Geometry: final body of the model. Coordinates: model frame, mm. Face numbers are marked on the shaded views. Give positions to 0.01 mm unless a question says otherwise; leave off trailing zeros. Put each result on its own line as item: value. Start each with the question number.
1. First-contact query: P1, Ø1.7, axis at x = 0.5, z = -20, coming from the -Y side; P2, Ø3.5, axis at x = 0, z = -19.05, coming from the +Y side. Flat tips, straight axial feed; report the tip coordinate or a pass-through.
2. Ray query, line 1 along Z through (x, y) = (0, -515.75); line 2 along X through (y, z) = (-19, -19); line 3 along X through (y, z) = (-352, -40.5). Return the intervals inside material, ascending. Write a range as from..to.
3. Mould query, pull axis Z, two halves, no side actions, for the marked faces 1, 2 and 3. Classes: pulls with the +Z half, pulls with the -Z half, needs draft (parallel to the pull), parting line crosses it, or undercut.
from build123d import *

# Parameters (mm, degrees)
F0_W     = 38.1
F0_H     = 88.9
F1_DEPTH = 533.4
F2_R     = 5.08
F3_R     = 2.8575
F4_DEPTH = 25.4
F5_R     = 2.8575
F6_DEPTH = 25.4


with BuildPart() as f1:
    # F0 (on Front) → F1 (new body)
    with BuildSketch(Plane.XZ):
        Rectangle(F0_W, F0_H)
    extrude(amount=F1_DEPTH)

    # F2
    f2_edges = [f1.edges().sort_by_distance(p)[0] for p in [
        (19.05, -266.7, 44.45),
        (-19.05, -266.7, 44.45),
        (19.05, -266.7, -44.45),
        (-19.05, -266.7, -44.45),
    ]]
    fillet(f2_edges, radius=F2_R)

    # F3 (on face) → F4 (cut)
    with BuildSketch(Plane.XZ.offset(533.4)):
        with Locations((0, -19.05)):
            Circle(F3_R)
        with Locations((0, 19.05)):
            Circle(F3_R)
    extrude(amount=-F4_DEPTH, mode=Mode.SUBTRACT)

    # F5 (on face) → F6 (cut)
    with BuildSketch(Plane(origin=(0, 0, 0), x_dir=(-1, 0, 0), z_dir=(0, 1, 0))):
        with Locations((0, 19.05)):
            Circle(F5_R)
        with Locations((0, -19.05)):
            Circle(F5_R)
    extrude(amount=-F6_DEPTH, mode=Mode.SUBTRACT)


solid = f1.part
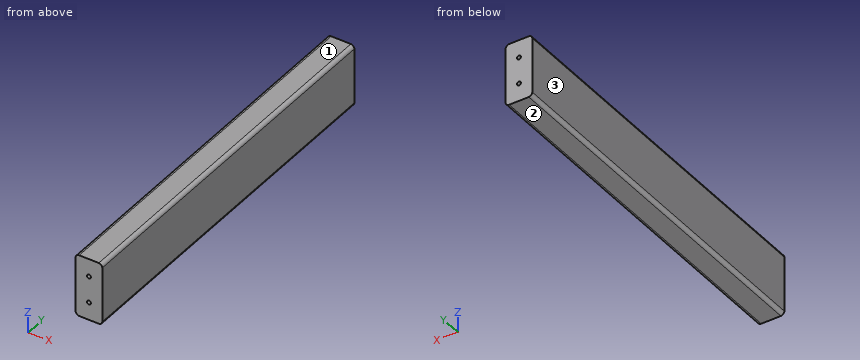
Resolved:
1. P1: y = -508
1. P2: y = -25.4
2. line 1: -44.45..-21.91, -16.19..16.19, 21.91..44.45
2. line 2: -19.05..-2.86, 2.86..19.05
2. line 3: -18.92..18.92
3. face 1: pulls with the +Z half
3. face 2: pulls with the -Z half
3. face 3: needs draft
